For this review, take the finished solid that the model builds, in its own axes (mm). A direction names the side the tool comes from. Coordinates: 2 decimals unless noted, no trailing zeros. Loops run counter-clockwise (first coordinate to the right, second up) from the corner with the lowest first, then second, coordinate; pieces in that order, holes last.
1. To check wall thickness, follow probe 1 along X at (y, z) = (160, 0.5); probe 2 along Y at (x, z) = (55, 0.4); probe 3 along Y at (x, z) = (9, 0.9). State the ranges of each line that lie inside material, in increasing order.
2. Take a section at B-B, the plane x = -26. State the section outline as (y, z) points.
3. Machinability: for faces 1 (the face through (48, 81, 1)), 2 (the face through (-1, 65, 1.5)), which of the approach directions +Z, -Z, +X, -X, +Y, -Y give a long, thin tool a straight path to every point of the face, cutting with its end or side? Answer none if there is none.
4. Clearance check with a flat-ended pin moving along its axis: P1, Ø1.8, axis at x = -55, y = 160, coming from the -Z side. State where the tip first meets the part, or that it passes through.
5. Mouldability with a two-part tool opening along X and no side actions: class faces 3 (the face through (-1, 65, 0)), 4 (the face through (-48, 81, 1)) as pulls with the +X half, pulls with the -X half, needs draft (parallel to the pull), parting line crosses it, or undercut.
6. Take a section at A-A, the plane z = 0.65. Count the separate pieces of the cut face and the enclosed holes in it, then the cut area to 3 significant figures.
```python
from build123d import *

# Parameters (mm, degrees)
ESQUISSE1_W             = 149
ESQUISSE1_H             = 165
ESQUISSE1_W_2           = 100
ESQUISSE1_H_2           = 55
BOSS_EXTRU_1_DEPTH      = 1.5
CONG_1_R                = 5
ESQUISSE2_R             = 1.5
ENL_V_MAT_EXTRU_1_DEPTH = 182.045574373


with BuildPart() as part:
    # Esquisse1 → Boss.-Extru.1 (new body)
    with BuildSketch(Plane.XY):
        with Locations((0, 82.5)):
            Rectangle(ESQUISSE1_W, ESQUISSE1_H)
        with Locations((0, 107.5)):
            Rectangle(ESQUISSE1_W_2, ESQUISSE1_H_2, mode=Mode.SUBTRACT)
    extrude(amount=BOSS_EXTRU_1_DEPTH)

    # Congé1
    cong_1_edges = [part.edges().sort_by_distance(p)[0] for p in [
        (-50, 135, 0.75),
        (-50, 80, 0.75),
        (50, 80, 0.75),
        (50, 135, 0.75),
    ]]
    fillet(cong_1_edges, radius=CONG_1_R)

    # Esquisse2 → Enlèv. mat.-Extru.1 (cut, through all)
    with BuildSketch(Plane.XY.offset(1.5)):
        with Locations((-30, 147.5)):
            Circle(ESQUISSE2_R)
        with Locations(Location((-30, 67.5, 0), (0, 0, 180))):
            Circle(ESQUISSE2_R)
        with Locations((30, 67.5)):
            Circle(ESQUISSE2_R)
        with Locations(Location((30, 147.5, 0), (0, 0, 180))):
            Circle(ESQUISSE2_R)
        with Locations((-55, 160)):
            Circle(ESQUISSE2_R)
        with Locations(Location((-55, 5, 0), (0, 0, 180))):
            Circle(ESQUISSE2_R)
        with Locations((55, 5)):
            Circle(ESQUISSE2_R)
        with Locations(Location((55, 160, 0), (0, 0, 180))):
            Circle(ESQUISSE2_R)
    extrude(amount=-ENL_V_MAT_EXTRU_1_DEPTH, mode=Mode.SUBTRACT)


solid = part.part
```
Results list:
1. probe 1: x = -74.5 to -56.5, -53.5 to 53.5, 56.5 to 74.5
1. probe 2: y = 0 to 3.5, 6.5 to 158.5, 161.5 to 165
1. probe 3: y = 0 to 80, 135 to 165
2. outline: (0, 0) - (80, 0) - (80, 1.5) - (0, 1.5) - close; (135, 0) - (165, 0) - (165, 1.5) - (135, 1.5) - close
3. face 1: +Z, -Z
3. face 2: +Z, +X, -X, +Y, -Y
4. P1: passes through
5. face 3: needs draft
5. face 4: undercut
6. separate pieces: 1
6. enclosed holes: 9
6. area: 19,000 mm2
